```python
from build123d import *

# Parameters (mm, degrees)
SKETCH_1_W          = 180
SKETCH_1_H          = 120
EXTRUDE_1_DEPTH     = 4
SKETCH_3_W          = 40
SKETCH_3_H          = 30
CUT_EXTRUDE_2_DEPTH = 4
SKETCH_4_R          = 1.6
CUT_EXTRUDE_3_DEPTH = 4
SKETCH_5_R          = 1.6
CUT_EXTRUDE_4_DEPTH = 4
SKETCH_7_R          = 2
CUT_EXTRUDE_5_DEPTH = 10


with BuildPart() as part:
    # 草图1 → 凸台-拉伸1 (new body)
    with BuildSketch(Plane(origin=(0, 0, 0), x_dir=(1, 0, 0), z_dir=(0, 1, 0))):
        Rectangle(SKETCH_1_W, SKETCH_1_H)
    extrude(amount=EXTRUDE_1_DEPTH)

    # 草图3 → 切除-拉伸2 (cut)
    with BuildSketch(Plane(origin=(0, 4, 0), x_dir=(1, 0, 0), z_dir=(0, 1, 0))):
        with Locations((80, 0)):
            Rectangle(SKETCH_3_W, SKETCH_3_H)
    extrude(amount=-CUT_EXTRUDE_2_DEPTH, mode=Mode.SUBTRACT)

    # 草图4 → 切除-拉伸3 (cut)
    with BuildSketch(Plane(origin=(0, 4, 0), x_dir=(1, 0, 0), z_dir=(0, 1, 0))):
        with Locations(Location((-17, 56, 0), (0, 0, 270))):
            Circle(SKETCH_4_R)
        with Locations(Location((20, 56, 0), (0, 0, 270))):
            Circle(SKETCH_4_R)
        with Locations(Location((20, 19, 0), (0, 0, 270))):
            Circle(SKETCH_4_R)
        with Locations(Location((-17, 19, 0), (0, 0, 270))):
            Circle(SKETCH_4_R)
    extrude(amount=-CUT_EXTRUDE_3_DEPTH, mode=Mode.SUBTRACT)

    # 草图5 → 切除-拉伸4 (cut)
    with BuildSketch(Plane(origin=(0, 4, 0), x_dir=(1, 0, 0), z_dir=(0, 1, 0))):
        with Locations(Location((-29.5, -7.8, 0), (0, 0, 270))):
            Circle(SKETCH_5_R)
        with Locations(Location((20, -23, 0), (0, 0, 270))):
            Circle(SKETCH_5_R)
        with Locations(Location((20, -50.9, 0), (0, 0, 270))):
            Circle(SKETCH_5_R)
        with Locations(Location((-30.8, -56, 0), (0, 0, 270))):
            Circle(SKETCH_5_R)
    extrude(amount=-CUT_EXTRUDE_4_DEPTH, mode=Mode.SUBTRACT)

    # 草图7 → 切除-拉伸5 (cut)
    with BuildSketch(Plane.XZ):
        with Locations(Location((52, 16, 0), (0, 0, 270))):
            Circle(SKETCH_7_R)
        with Locations(Location((38, 16, 0), (0, 0, 270))):
            Circle(SKETCH_7_R)
        with Locations(Location((52, -16, 0), (0, 0, 270))):
            Circle(SKETCH_7_R)
        with Locations(Location((38, -16, 0), (0, 0, 270))):
            Circle(SKETCH_7_R)
    extrude(amount=-CUT_EXTRUDE_5_DEPTH, mode=Mode.SUBTRACT)


solid = part.part
```
Check sheet for the modelled part. Datum: model origin and axes. Units: mm. A direction names the side the tool comes from. Round coordinates to 2 decimals unless told otherwise and drop trailing zeros. Loops run counter-clockwise (first coordinate to the right, second up) from the corner with the lowest first, then second, coordinate; pieces in that order, holes last. Notation, with made-up numbers: (40, 39) - (69, 39) arc R31 ccw to (69, 70) - close; hole circle Ø9 at (45.25, 86). An arc over 180 degrees is marked (long way). Answer as a JSON object with one key per item and string values. Group by question number.
Q1. Scan lines: line 1 along X through (y, z) = (2.2, 16); line 2 along X through (y, z) = (2.9, 50.9); line 3 along Z through (x, y) = (80, 0.9). Record each from-to range of solid material in increasing order. Write a range as [from, to].
Q2. Sectioned sample at B-B, the plane y = 1.9. Count the separate pieces of the cut face and the enclosed holes in it, plus the area to 3 significant figures.
Q3. Mould release check, pull along Z, two halves, no side actions. Record for faces 1 (the face through (90, 2, -37)), 2 (the face through (-1, 2, 60)), 3 (the face through (36.226, 1.972, -16.923)): released by +Z, released by -Z, zero draft, split by the parting line, or undercut.
Q4. Set-up check for faces 4 (the face through (75, 2, -15)), 5 (the face through (-1, 2, -60)): record each of +Z, -Z, +X, -X, +Y, -Y from which the full face is reachable in a straight line by a thin tool's end or side.
Q5. Sectioned sample at A-A, the plane x = 66.5. Enter the section's corners in (y, z).
Solution:
{
 "1": {"line 1": "x = [-90, 36], [40, 50], [54, 90]", "line 2": "x = [-90, 18.4], [21.6, 90]", "line 3": "z = [-60, -15], [15, 60]"},
 "2": {"separate pieces": "1", "enclosed holes": "12", "area": "20,600 mm²"},
 "3": {"face 1": "zero draft", "face 2": "released by +Z", "face 3": "undercut"},
 "4": {"face 4": "+X, +Y, -Y", "face 5": "-Z, +X, -X, +Y, -Y"},
 "5": {"outline": "(0, -60) - (4, -60) - (4, -15) - (0, -15) - close; (0, 15) - (4, 15) - (4, 60) - (0, 60) - close"}
}
